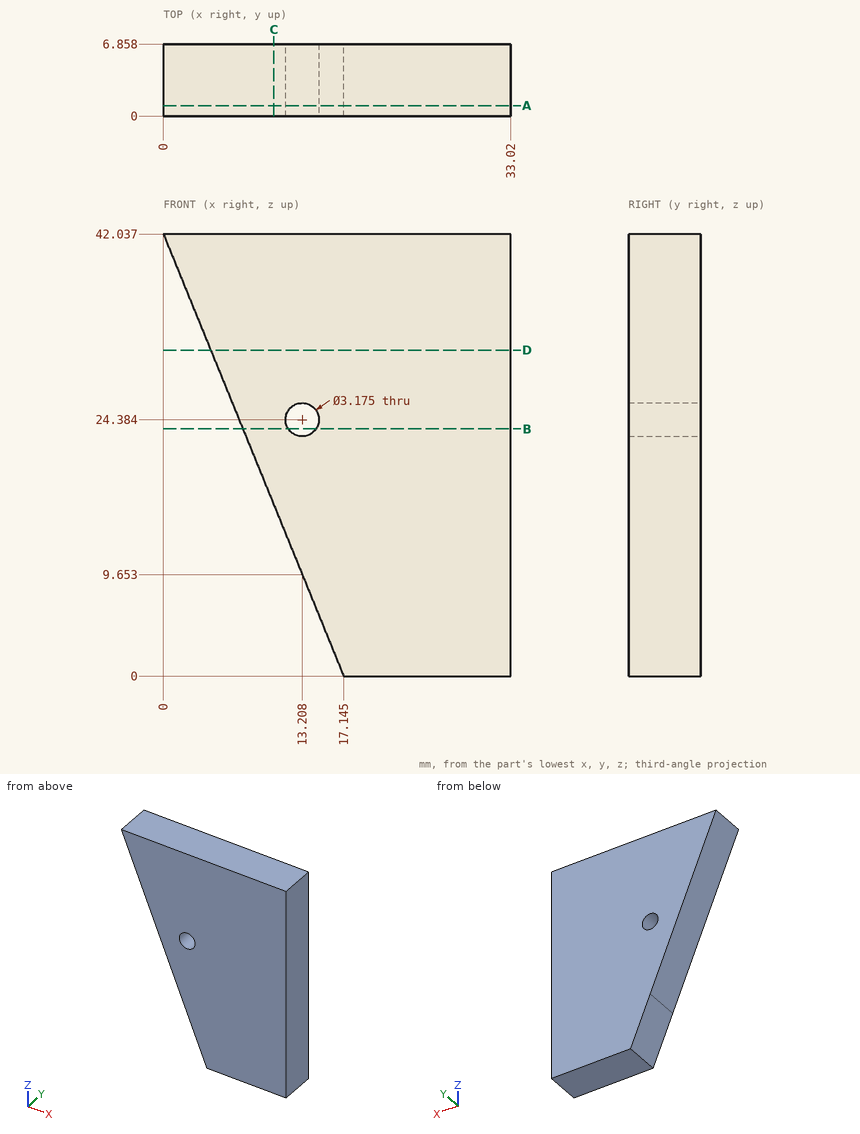
The figure shows three views and two pictorial views of one solid part (mm, origin at its lowest corner). Answer the questions. Round coordinates to 2 decimals unless told otherwise and drop trailing zeros. Loops run counter-clockwise (first coordinate to the right, second up) from the corner with the lowest first, then second, coordinate; pieces in that order, holes last. Notation, with made-up numbers: (23.25, 60) - (61.25, 60) arc R16 ccw to (61.25, 76) - close; hole circle Ø2 at (1, 8). An arc over 180 degrees is marked (long way). Use one line per item in the form item = value. Start each with the question number.
(1) Find section B-B on z = 23.5. Determine the outline of the cut face in (x, y), and give its area (3 significant figures).
(2) Find section A-A on y = 1. Determine the outline of the cut face in (x, z) (1 decimal), and give its area (3 significant figures).
(3) Consider line 1 (X direction, y = 4.25, z = 25.5) (1 decimal); line 2 (Z direction, x = 16, y = 4.5); line 3 (X direction, y = 5, z = 19). Determine where each line is inside the solid, lowest interval first.
(4) Flat-ended cylindrical pins translate along their axes: P1, Ø1.9, axis at x = 13.208, z = 24.384, coming from the -Y side; P2, Ø1, axis at x = 12, z = 34.5, coming from the -Y side. Find the tip coordinate at first contact, or state that the pin passes through.
(5) Find section D-D on z = 31. Determine the outline of the cut face in (x, y).
(6) Find section C-C on x = 10.5. Determine the outline of the cut face in (y, z), and give its area (3 significant figures).
Answer list:
q1.outline = (7.56, 0) - (11.89, 0) - (11.89, 6.86) - (7.56, 6.86) - close; (14.53, 0) - (33.02, 0) - (33.02, 6.86) - (14.53, 6.86) - close
q1.area = 157 mm^2
q2.outline = (0, 42) - (17.1, 0) - (33, 0) - (33, 42) - close; hole circle Ø3.2 at (13.2, 24.4)
q2.area = 1,020 mm^2
q3.line_1 = 6.7 to 12.1, 14.3 to 33
q3.line_2 = 2.81 to 42.04
q3.line_3 = 9.4 to 33.02
q4.P1 = through
q4.P2 = 0
q5.outline = (4.5, 0) - (33.02, 0) - (33.02, 6.86) - (4.5, 6.86) - close
q6.outline = (0, 16.29) - (6.86, 16.29) - (6.86, 42.04) - (0, 42.04) - close
q6.area = 177 mm^2
